The model under review builds one solid part; all positions refer to its coordinate system, in mm. Coordinates: 2 decimals unless noted, no trailing zeros. Order: outer loops, then holes, each group sorted by start corner. A loop starts at its lowest first (then second) coordinate and runs counter-clockwise, first axis right, second up. Notation, with made-up numbers: (21, 49) -> (80, 49) arc R29 cw to (80, 88) -> close; hole circle Ø11 at (3.5, 18). An arc over 180 degrees is marked (long way). Use one line per item in the form item = value. Start each with the question number.
(1) Mouldability with a two-part tool opening along Z and no side actions: class faces 1 (the flat face through (0, 0, 0)), 2 (the flat face through (0, 31.5, 0)), 3 (the cylindrical face through (9.568, 15.558, -1.256)) as +Z half, -Z half, draft (parallel to the pull), parting line (faces both ways), or undercut.
(2) Wall thickness on line 1 along Y through (x, z) = (2, 7.5); line 2 along X through (y, z) = (26, 0); line 3 along Y through (x, z) = (7, -6.25): over which ranges is each line inside the solid? List them lowest first.
(3) Insertion check: pin 1 Ø8 at (y, z) = (7.5, -4.5) entering from -X; pin 2 Ø5 at (y, z) = (7, 7) entering from +X; pin 3 Ø1 at (x, y) = (4, 19) entering from +Z. Each pin has a flat end and moves straight along its axis. Give the tip position at first contact, or say it passes through.
(4) Take a section at A-A (y = 17). State the section outline as (x, z) points.
```python
from build123d import *

# Parameters (mm, degrees)
SKETCH1_R           = 9.65
BOSS_EXTRUDE1_DEPTH = 31.5
FILLET4_R           = 2
SKETCH2_R           = 0.35
BOSS_EXTRUDE2_DEPTH = 0.1
CIRPATTERN1_COUNT   = 14


with BuildPart() as part:
    # Sketch1 → Boss-Extrude1 (new body)
    with BuildSketch(Plane(origin=(0, 0, 0), x_dir=(1, 0, 0), z_dir=(0, 1, 0))):
        with Locations(Location((0, 0, 0), (0, 0, 270))):
            Circle(SKETCH1_R)
    extrude(amount=BOSS_EXTRUDE1_DEPTH)

    # Fillet4
    fillet4_edges = [part.edges().sort_by_distance(p)[0] for p in [
        (0, 0, -9.65),
        (0, 31.5, -9.65),
    ]]
    fillet(fillet4_edges, radius=FILLET4_R)

    # Sketch2 → Boss-Extrude2 (add)
    with BuildSketch(Plane(origin=(0, 31.5, 0), x_dir=(1, 0, 0), z_dir=(0, 1, 0))):
        with Locations(Location((0, 6, 0), (0, 0, 270))):
            Circle(SKETCH2_R)
    boss_extrude2 = extrude(amount=BOSS_EXTRUDE2_DEPTH)

    # CirPattern1: Boss-Extrude2 ×14 about axis
    cirpattern1_axis = Axis((0, 0, 0), (0, 1, 0))
    for i in range(1, CIRPATTERN1_COUNT):
        add(boss_extrude2.rotate(cirpattern1_axis, i * 360 / CIRPATTERN1_COUNT))


solid = part.part
```
Findings:
q1.face_1 = draft
q1.face_2 = undercut
q1.face_3 = parting line
q2.line_1 = 0 to 31.5
q2.line_2 = -9.65 to 9.65
q2.line_3 = 1 to 30.5
q3.pin_1 = -9.64
q3.pin_2 = 8.54
q3.pin_3 = 8.99
q4.outline = circle Ø19.3 at (0, 0)
